```python
from build123d import *

# Parameters (mm, degrees)
CUT_EXTRUDE1_START  = -28.722813
SKETCH2_OUTSIDE_W   = 96.248
SKETCH2_OUTSIDE_H   = 96.248
CUT_EXTRUDE1_DEPTH  = 57.445626
BOSS_EXTRUDE1_DEPTH = 36
SKETCH4_R           = 3.5
CUT_EXTRUDE2_DEPTH  = 5
LPATTERN1_COUNT     = 2
LPATTERN1_PITCH     = 35
BOSS_EXTRUDE2_DEPTH = 30
BOSS_EXTRUDE2_DRAFT = -7
BOSS_EXTRUDE6_DEPTH = 35
BOSS_EXTRUDE9_DEPTH = 30
BOSS_EXTRUDE9_DRAFT = 7
SKETCH10_R          = 25
BOSS_EXTRUDE7_DEPTH = 2
SKETCH11_R          = 3.5
BOSS_EXTRUDE8_DEPTH = 5
FILLET3_R           = 100


with BuildPart() as part:
    # Sketch1 → Revolve2 (revolve)
    with BuildSketch(Plane(origin=(0, 0, 0), x_dir=(1, 0, 0), z_dir=(0, 1, 0))):
        with BuildLine():
            Line((0, 35), (0, -35))
            ThreePointArc((0, -35), (35, 0), (0, 35))
        make_face()
    revolve(axis=Axis((0, 0, -35), (0, 0, 1)))

    # Sketch2 outside → Cut-Extrude1 (cut)
    with BuildSketch(Plane(origin=(0, 0, 0), x_dir=(1, 0, 0), z_dir=(0, 1, 0)).offset(CUT_EXTRUDE1_START)):
        Rectangle(SKETCH2_OUTSIDE_W, SKETCH2_OUTSIDE_H)
        with BuildLine():
            Line((-20, -28.722813233), (-20, 28.722813233))
            ThreePointArc((-20, 28.722813233), (0, 35), (20, 28.722813233))
            Line((20, 28.722813233), (20, -28.722813233))
            ThreePointArc((20, -28.722813233), (0, -35), (-20, -28.722813233))
        make_face(mode=Mode.SUBTRACT)
    extrude(amount=CUT_EXTRUDE1_DEPTH, mode=Mode.SUBTRACT)

    # Sketch3 → Boss-Extrude1 (add)
    with BuildSketch(Plane(origin=(0, 0, 0), x_dir=(1, 0, 0), z_dir=(0, 1, 0))):
        with BuildLine():
            Line((-20, 15), (-20, -15))
            ThreePointArc((-20, -15), (0, -25), (20, -15))
            Line((20, -15), (20, 15))
            ThreePointArc((20, 15), (0, 25), (-20, 15))
        make_face()
    extrude(amount=BOSS_EXTRUDE1_DEPTH)

    # Sketch4 → Cut-Extrude2 (cut)
    with BuildSketch(Plane.ZY.offset(20)):
        Circle(SKETCH4_R)
    cut_extrude2 = extrude(amount=-CUT_EXTRUDE2_DEPTH, mode=Mode.SUBTRACT)

    # LPattern1: Cut-Extrude2 ×2
    with Locations(*[(i * LPATTERN1_PITCH, 0, 0) for i in range(1, LPATTERN1_COUNT)]):
        add(cut_extrude2, mode=Mode.SUBTRACT)


with BuildPart() as boss_extrude2_tool:
    # Sketch5 → Boss-Extrude2 (with draft: the straight prism first)
    with BuildSketch(Plane(origin=(0, 36, 0), x_dir=(1, 0, 0), z_dir=(0, 1, 0))):
        with BuildLine():
            Line((-20, 15), (-20, 11.357816692))
            ThreePointArc((-20, 11.357816692), (-23, 0), (-20, -11.357816692))
            Line((-20, -11.357816692), (-20, -15))
            ThreePointArc((-20, -15), (0, -25), (20, -15))
            Line((20, -15), (20, -11.357816692))
            ThreePointArc((20, -11.357816692), (23, 0), (20, 11.357816692))
            Line((20, 11.357816692), (20, 15))
            ThreePointArc((20, 15), (0, 25), (-20, 15))
        make_face()
    extrude(amount=BOSS_EXTRUDE2_DEPTH)
    # Boss-Extrude2: the draft: its side faces are tilted about the plane it starts from
    boss_extrude2_sides = [boss_extrude2_tool.faces().sort_by_distance(p)[0] for p in [
        (20, 51, -13.178908346),
        (0, 51, -25),
        (-20, 51, -13.178908346),
        (-23, 51, 0),
        (-20, 51, 13.178908346),
        (0, 51, 25),
        (20, 51, 13.178908346),
        (23, 51, 0),
    ]]
    draft(boss_extrude2_sides, Plane(origin=(0, 36, 0), x_dir=(1, 0, 0), z_dir=(0, 1, 0)), BOSS_EXTRUDE2_DRAFT)


with BuildPart() as part_1:
    add(part.part)

    # Boss-Extrude2: add boss_extrude2_tool
    add(boss_extrude2_tool.part)

    # Sketch9 → Boss-Extrude6 (add)
    with BuildSketch(Plane(origin=(0, 66, 0), x_dir=(1, 0, 0), z_dir=(0, 1, 0))):
        with BuildLine():
            Line((23.683536827, 12.29232366), (23.683536827, 16.181327766))
            ThreePointArc((23.683536827, 16.181327766), (0, 28.683536827), (-23.683536827, 16.181327766))
            Line((-23.683536827, 16.181327766), (-23.683536827, 12.29232366))
            ThreePointArc((-23.683536827, 12.29232366), (-26.683536827, 0), (-23.683536827, -12.29232366))
            Line((-23.683536827, -12.29232366), (-23.683536827, -16.181327766))
            ThreePointArc((-23.683536827, -16.181327766), (0, -28.683536827), (23.683536827, -16.181327766))
            Line((23.683536827, -16.181327766), (23.683536827, -12.29232366))
            ThreePointArc((23.683536827, -12.29232366), (26.683536827, 0), (23.683536827, 12.29232366))
        make_face()
    extrude(amount=BOSS_EXTRUDE6_DEPTH)


with BuildPart() as boss_extrude9_tool:
    # Sketch12 → Boss-Extrude9 (with draft: the straight prism first)
    with BuildSketch(Plane(origin=(0, 101, 0), x_dir=(1, 0, 0), z_dir=(0, 1, 0))):
        with BuildLine():
            Line((23.683536827, 12.29232366), (23.683536827, 16.181327766))
            ThreePointArc((23.683536827, 16.181327766), (0, 28.683536827), (-23.683536827, 16.181327766))
            Line((-23.683536827, 16.181327766), (-23.683536827, 12.29232366))
            ThreePointArc((-23.683536827, 12.29232366), (-26.683536827, 0), (-23.683536827, -12.29232366))
            Line((-23.683536827, -12.29232366), (-23.683536827, -16.181327766))
            ThreePointArc((-23.683536827, -16.181327766), (0, -28.683536827), (23.683536827, -16.181327766))
            Line((23.683536827, -16.181327766), (23.683536827, -12.29232366))
            ThreePointArc((23.683536827, -12.29232366), (26.683536827, 0), (23.683536827, 12.29232366))
        make_face()
    extrude(amount=BOSS_EXTRUDE9_DEPTH)
    # Boss-Extrude9: the draft: its side faces are tilted about the plane it starts from
    boss_extrude9_sides = [boss_extrude9_tool.faces().sort_by_distance(p)[0] for p in [
        (0, 116, 28.683536827),
        (23.683536827, 116, 14.236825713),
        (26.683536827, 116, 0),
        (23.683536827, 116, -14.236825713),
        (0, 116, -28.683536827),
        (-23.683536827, 116, -14.236825713),
        (-26.683536827, 116, 0),
        (-23.683536827, 116, 14.236825713),
    ]]
    draft(boss_extrude9_sides, Plane(origin=(0, 101, 0), x_dir=(1, 0, 0), z_dir=(0, 1, 0)), BOSS_EXTRUDE9_DRAFT)


with BuildPart() as part_2:
    add(part_1.part)

    # Boss-Extrude9: add boss_extrude9_tool
    add(boss_extrude9_tool.part)

    # Sketch10 → Boss-Extrude7 (add)
    with BuildSketch(Plane(origin=(0, 131, 0), x_dir=(1, 0, 0), z_dir=(0, 1, 0))):
        with Locations(Location((0, 0, 0), (0, 0, 36.869897646))):
            Circle(SKETCH10_R)
    extrude(amount=BOSS_EXTRUDE7_DEPTH)

    # Sketch11 → Boss-Extrude8 (add)
    with BuildSketch(Plane(origin=(0, 133, 0), x_dir=(1, 0, 0), z_dir=(0, 1, 0))):
        with Locations(Location((0, 0, 0), (0, 0, 270))):
            Circle(SKETCH11_R)
    extrude(amount=BOSS_EXTRUDE8_DEPTH)

    # Fillet3
    # the kernel refuses this fillet: 100 mm, written as the material it takes off along each edge
    with BuildSketch(Plane(origin=(0, 66, 0), x_dir=(0.9978245122586105, 0, -0.06592603989218485), z_dir=(0.06592603989218485, 0, 0.9978245122586105))) as fillet3_piece_1:
        with BuildLine():
            CenterArc((28.683536827 - FILLET3_R, FILLET3_R * 0.0611626201505), FILLET3_R, 353, 7)
            Line((28.683536827, FILLET3_R * 0.0611626201505), (28.683536827, 0))
            Line((28.683536827, 0), (28.683536827 - FILLET3_R * 0.00745384835868, -FILLET3_R * 0.0607067232547))
        make_face()
    revolve(axis=Axis((0, 66, 0), (0, 1, 0)), revolution_arc=172.439949247, mode=Mode.SUBTRACT)
    with BuildSketch(Plane(origin=(0, 101, 0), x_dir=(0.9978245122586106, 0, -0.06592603989218539), z_dir=(0.06592603989218539, 0, 0.9978245122586106))) as fillet3_piece_2:
        with BuildLine():
            CenterArc((28.683536827 - FILLET3_R, -FILLET3_R * 0.0611626201505), FILLET3_R, 0, 7)
            Line((28.683536827 - FILLET3_R * 0.00745384835868, FILLET3_R * 0.0607067232547), (28.683536827, 0))
            Line((28.683536827, 0), (28.683536827, -FILLET3_R * 0.0611626201505))
        make_face()
    revolve(axis=Axis((0, 101, 0), (0, 1, 0)), revolution_arc=172.439949247, mode=Mode.SUBTRACT)
    with BuildSketch(Plane(origin=(0, 101, 0), x_dir=(-0.9978245122586106, 0, 0.06592603989218528), z_dir=(-0.06592603989218528, 0, -0.9978245122586106))) as fillet3_piece_3:
        with BuildLine():
            CenterArc((28.683536827 - FILLET3_R, -FILLET3_R * 0.0611626201505), FILLET3_R, 0, 7)
            Line((28.683536827 - FILLET3_R * 0.00745384835868, FILLET3_R * 0.0607067232547), (28.683536827, 0))
            Line((28.683536827, 0), (28.683536827, -FILLET3_R * 0.0611626201505))
        make_face()
    revolve(axis=Axis((0, 101, 0), (0, 1, 0)), revolution_arc=172.439949247, mode=Mode.SUBTRACT)
    with BuildSketch(Plane(origin=(0, 66, 0), x_dir=(-0.9978245122586105, 0, 0.06592603989218485), z_dir=(-0.06592603989218485, 0, -0.9978245122586105))) as fillet3_piece_4:
        with BuildLine():
            CenterArc((28.683536827 - FILLET3_R, FILLET3_R * 0.0611626201505), FILLET3_R, 353, 7)
            Line((28.683536827, FILLET3_R * 0.0611626201505), (28.683536827, 0))
            Line((28.683536827, 0), (28.683536827 - FILLET3_R * 0.00745384835868, -FILLET3_R * 0.0607067232547))
        make_face()
    revolve(axis=Axis((0, 66, 0), (0, 1, 0)), revolution_arc=172.439949247, mode=Mode.SUBTRACT)


solid = part_2.part
```
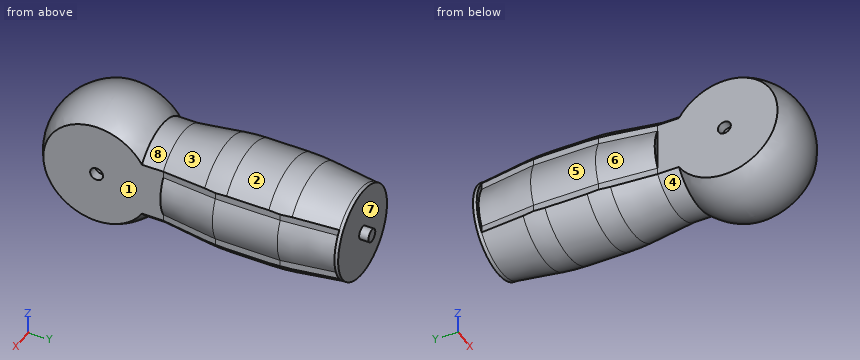
Geometry check sheet. Reference: the model listing, model coordinates, mm. Face numbers are marked on the shaded views. A direction names the side the tool comes from. Give positions to 0.01 mm unless a question says otherwise; leave off trailing zeros. Loops run counter-clockwise (first coordinate to the right, second up) from the corner with the lowest first, then second, coordinate; pieces in that order, holes last. Notation, with made-up numbers: M -2.5,70 L 47.5,70 A17 cw 47.5,79 Z; hole C 77.5,40 d3. An arc over 180 degrees is marked long. Write item = value, one per line. Start each with the question number.
1. Section check C-C, the plane y = 119.5. Enter the section's corners in (x, z), plus the area to 3 significant figures.
2. Thickness scan on probe 1 along Z at (x, y) = (-14, 88.5); probe 2 along Y at (x, z) = (21, -8); probe 3 along X at (y, z) = (-10, -13.5). Record the ranges inside material, lowest first.
3. Section check A-A, the plane y = 0. Enter the section's corners in (x, z).
4. Section check B-B, the plane y = 26.5. Enter the section's corners in (x, z), plus the area to 3 significant figures.
5. Tool access check on the marked faces 1, 2, 3 and 4. Record the directions out of +Z, -Z, +X, -X, +Y, -Y that give a thin tool (end or side, any length) a straight path to the whole face; none if there is none.
6. Draft check along Y on the marked faces 5, 6, 7 and 8. Enter one of: +Y half, -Y half, draft (parallel to the pull), parting line (faces both ways), or undercut.
7. Go/stop test with flat-tipped pins: P1, Ø2, axis at y = -1.5, z = 0.5, coming from the +X side; P2, Ø3.5, axis at x = 21, z = 1.5, coming from the -Y side; P3, Ø3.5, axis at y = -1.5, z = 0, coming from the -X side. Record where each tip stops, or that it passes through.
Values follow:
q1.outline = M -21.41,-15.46 A26.41 ccw 21.41,-15.46 L 21.41,-11.72 A24.41 ccw 21.41,11.72 L 21.41,15.46 A26.41 ccw -21.41,15.46 L -21.41,11.72 A24.41 ccw -21.41,-11.72 Z
q1.area = 2,080 mm^2
q2.probe_1 = -25.03 to 25.03
q2.probe_2 = 36 to 133
q2.probe_3 = -20 to 20
q3.outline = M -20,-28.72 A35 ccw 20,-28.72 L 20,-3.5 L 15,-3.5 L 15,3.5 L 20,3.5 L 20,28.72 A35 ccw -20,28.72 L -20,3.5 L -15,3.5 L -15,-3.5 L -20,-3.5 Z
q4.outline = M -20,-15 A25 ccw 20,-15 L 20,15 A25 ccw -20,15 Z
q4.area = 1,760 mm^2
q5.face_1 = +Z, -Z, +X, -Y
q5.face_2 = +Z, +Y
q5.face_3 = +Z
q5.face_4 = -Z
q6.face_5 = draft
q6.face_6 = -Y half
q6.face_7 = +Y half
q6.face_8 = undercut
q7.P1 = 15
q7.P2 = -29.2
q7.P3 = -15
